Source: CAD feature listing. Evaluate the final solid. Frame: model axes, mm. Round coordinates to 2 decimals unless told otherwise and drop trailing zeros. Write each loop counter-clockwise with the first axis right and the second up, starting at its lowest first coordinate (ties: lowest second). Pieces come first, ordered by that corner, then holes. Notation, with made-up numbers: M 10.5,30.25 L 48.5,30.25 A24 cw 48.5,68.25 Z; hole C 33.5,34 d7. An arc over 180 degrees is marked long. Answer in a Markdown table with one row per item.
from build123d import *

# Parameters (mm, degrees)
SKETCH240_R             = 4.5
SKETCH240_R_2           = 2.5
PAD102_DEPTH            = 11
SKETCH241_R             = 1.5
POCKET047_DEPTH         = 5
SKETCH242_R             = 1.6
FILLET_R                = 0.5
BODY010_PLACEMENT_ANGLE = 90


with BuildPart() as part:
    # Sketch240 → Pad102 (new body)
    with BuildSketch(Plane.XZ):
        Circle(SKETCH240_R)
        Circle(SKETCH240_R_2, mode=Mode.SUBTRACT)
    extrude(amount=PAD102_DEPTH)

    # Sketch241 (on DatumPlane) → Pocket047 (cut)
    with BuildSketch(Plane.XY.offset(5)):
        with Locations((0, -1.9)):
            Circle(SKETCH241_R)
    extrude(amount=-POCKET047_DEPTH, mode=Mode.SUBTRACT)

    # Sketch242 (on DatumPlane) → Groove (revolve, cut)
    with BuildSketch(Plane.XY):
        with Locations((5, -8)):
            Circle(SKETCH242_R)
    revolve(axis=Axis((0, 0, 0), (0, 1, 0)), mode=Mode.SUBTRACT)

    # Fillet
    fillet_edges = [part.edges().sort_by_distance(p)[0] for p in [
        (-4.5, -9.519868, 0),
        (-4.5, -6.480132, 0),
    ]]
    fillet(fillet_edges, radius=FILLET_R)


with BuildPart() as part_1:
    # Body010 placement: moved
    add(part.part.moved(Location((15.12, 4.94, 111.21))).rotate(Axis((15.12, 4.94, 111.21), (0, 0, 1)), BODY010_PLACEMENT_ANGLE))


solid = part_1.part
Q1. Contact query for flat-ended pins moving along their axis: pin 1 Ø1.5 at (x, y) = (23.5, 7) entering from +Z; pin 2 Ø4.5 at (y, z) = (4.94, 111.21) entering from +X; pin 3 Ø5 at (x, z) = (22, 114.5) entering from +Y. Output: stop coordinate, or through.
Solutions:
| item | result |
|---|---|
| pin 1 | stops at z = 114.59 |
| pin 2 | passes through |
| pin 3 | stops at y = 9.35 |
Q2. Pull-direction query (X, two-part tool) for faces 1 (the cylindrical face through (16.57, 6.37, 114.48)), 2 (the flat face through (26.12, 7, 109)), 3 (the flat face through (15.12, 7, 109)); classes: pulls with the +X half, pulls with the -X half, needs draft (parallel to the pull), parting line crosses it, or undercut.
Solutions:
| item | result |
|---|---|
| face 1 | undercut |
| face 2 | pulls with the +X half |
| face 3 | pulls with the -X half |
Q3. Section D-D (x = 17.02). Return loops of the section in (y, z), and give its area (3 significant figures).
Solutions:
| item | result |
|---|---|
| outline | M 3.44,113.21 L 3.44,115.45 A4.5 ccw long 6.44,115.45 L 6.44,113.21 A2.5 cw long Z |
| area | 37.8 mm2 |
Q4. Material intervals for probe 1 along Z at (x, y) = (19.25, 4.94); probe 2 along X at (y, z) = (4.94, 114); probe 3 along Y at (x, z) = (16.5, 115), sorted ascending.
Solutions:
| item | result |
|---|---|
| probe 1 | z = 106.71 to 108.71, 113.71 to 115.71 |
| probe 2 | x = 15.12 to 15.52, 18.52 to 26.12 |
| probe 3 | y = 2.51 to 3.53, 6.35 to 7.37 |
Q5. Section A-A (y = 4.94). State how many separate pieces and enclosed holes the cut face has, and give its area (3 significant figures).
Solutions:
| item | result |
|---|---|
| separate pieces | 3 |
| enclosed holes | 0 |
| area | 33.0 mm2 |
Q6. Section C-C (x = 20). Return loops of the section in (y, z), and give its area (3 significant figures).
Solutions:
| item | result |
|---|---|
| outline | C 4.94,111.21 d9; hole C 4.94,111.21 d5 |
| area | 44.0 mm2 |
